Here's how the part is built. I have some questions about the finished solid (model axes, mm). A direction names the side the tool comes from. Give positions to 0.01 mm unless a question says otherwise; leave off trailing zeros. Loops run counter-clockwise (first coordinate to the right, second up) from the corner with the lowest first, then second, coordinate; pieces in that order, holes last. Notation, with made-up numbers: (16.5, 14.25) - (63.5, 14.25) arc R23 ccw to (63.5, 37.25) - close; hole circle Ø11 at (13, 53.25). An arc over 180 degrees is marked (long way). Use a Markdown table: item, result.
from build123d import *

# Parameters (mm, degrees)
SKETCH_1_W                         = 560
SKETCH_1_H                         = 90
SM_BASE_FLANGE_1_DEPTH             = 3
SM_EDGE_FLANGE_4_DEPTH             = 560
SM_START                           = 3
SM_EDGE_FLANGE_4_FLAT_DEPTH        = 3
SM_EDGE_FLANGE_4_BEND_DEPTH        = 560
SM_EDGE_FLANGE_4_FLAT_2_DEPTH      = 3
SM_EDGE_FLANGE_5_STRIP_W           = 13.4732
SM_EDGE_FLANGE_5_STRIP_H           = 3
SM_EDGE_FLANGE_5_STRIP_CUT_DEPTH   = 460
SM_EDGE_FLANGE_5_STRIP_2_W         = 13.4732
SM_EDGE_FLANGE_5_STRIP_2_H         = 3
SM_EDGE_FLANGE_5_STRIP_CUT_2_DEPTH = 460
SM_EDGE_FLANGE_5_DEPTH             = 460
SM_EDGE_FLANGE_5_BEND_DEPTH        = 460
FILLET_2_R                         = 5
HOLE_WIZARD_M6_1_D                 = 5
HOLE_WIZARD_M6_1_DEPTH             = 3
HOLE_WIZARD_M6_1_2_D               = 6.6
HOLE_WIZARD_M6_1_2_DEPTH           = 3
SKETCH_62_R                        = 10
SKETCH_62_R_2                      = 6
CUT_EXTRUDE_1_DEPTH                = 10
FILLET_3_R                         = 3
HOLE_WIZARD_M8_1_D                 = 9
SM_START_2                         = -44.7366
SM_EDGE_FLANGE_6_DEPTH             = 89.4732
SM_START_3                         = -45
SM_EDGE_FLANGE_6_2_DEPTH           = 90
SM_START_4                         = -283.7366
SM_EDGE_FLANGE_6_3_DEPTH           = 3
CUT_EXTRUDE_2_REACH                = 323.451
SKETCH_69_R                        = 6
CUT_EXTRUDE_3_REACH                = 333.07
FILLET_4_R                         = 3


with BuildPart() as part:
    # 베이스-플랜지1: sheet metal written as solids
    # Sketch 1 → 베이스-플랜지1 (new body)
    with BuildSketch(Plane(origin=(0, 0, 0), x_dir=(1, 0, 0), z_dir=(0, 1, 0))):
        Rectangle(SKETCH_1_W, SKETCH_1_H)
    extrude(amount=-SM_BASE_FLANGE_1_DEPTH)

    # 모서리 플랜지4: sheet metal written as solids
    # 모서리 플랜지4 bend section (on a plane across the edge) → 모서리 플랜지4 (add)
    with BuildSketch(Plane(origin=(-280, 0, 45.7366), x_dir=(0, 0, -1), z_dir=(1, 0, 0))):
        with BuildLine():
            Line((-3, 0.7366), (0, 0.7366))
            ThreePointArc((0, 0.7366), (0.215745145, 0.215745145), (0.7366, 0))
            Line((0.7366, 0), (0.7366, -3))
            ThreePointArc((0.7366, -3), (-1.905575199, -1.905575199), (-3, 0.7366))
        make_face()
    extrude(amount=SM_EDGE_FLANGE_4_DEPTH)

    # 모서리 플랜지4 profile (on flange) → 모서리 플랜지4 flat (add)
    with BuildSketch(Plane.XY.offset(45.7366).offset(SM_START)):
        Polygon((-280, 140), (-280, 0.7366), (280, 0.7366), (280, 20), (180, 20), (180, 140), align=None)
    extrude(amount=-SM_EDGE_FLANGE_4_FLAT_DEPTH)

    # 모서리 플랜지4 bend section 2 (on a plane across the edge) → 모서리 플랜지4 bend (add)
    with BuildSketch(Plane(origin=(280, 0, -45.7366), x_dir=(0, 0, 1), z_dir=(-1, 0, 0))):
        with BuildLine():
            Line((-3, 0.7366), (0, 0.7366))
            ThreePointArc((0, 0.7366), (0.215745145, 0.215745145), (0.7366, 0))
            Line((0.7366, 0), (0.7366, -3))
            ThreePointArc((0.7366, -3), (-1.905575199, -1.905575199), (-3, 0.7366))
        make_face()
    extrude(amount=SM_EDGE_FLANGE_4_BEND_DEPTH)

    # 모서리 플랜지4 profile 2 (on flange) → 모서리 플랜지4 flat 2 (add)
    with BuildSketch(Plane(origin=(0, 0, -45.7366), x_dir=(-1, 0, 0), z_dir=(0, 0, -1)).offset(SM_START)):
        Polygon((-280, 20), (-280, 0.7366), (280, 0.7366), (280, 140), (-180, 140), (-180, 20), align=None)
    extrude(amount=-SM_EDGE_FLANGE_4_FLAT_2_DEPTH)

    # 모서리 플랜지5: sheet metal written as solids
    # 모서리 플랜지5 strip (on a plane across the edge) → 모서리 플랜지5 strip cut (cut)
    with BuildSketch(Plane(origin=(-280, 140, 45.7366), x_dir=(0, -1, 0), z_dir=(1, 0, 0))):
        with Locations((-3, -1.5)):
            Rectangle(SM_EDGE_FLANGE_5_STRIP_W, SM_EDGE_FLANGE_5_STRIP_H)
    extrude(amount=SM_EDGE_FLANGE_5_STRIP_CUT_DEPTH, mode=Mode.SUBTRACT)

    # 모서리 플랜지5 strip 2 (on a plane across the edge) → 모서리 플랜지5 strip cut 2 (cut)
    with BuildSketch(Plane(origin=(180, 140, -45.7366), x_dir=(0, -1, 0), z_dir=(-1, 0, 0))):
        with Locations((-3, -1.5)):
            Rectangle(SM_EDGE_FLANGE_5_STRIP_2_W, SM_EDGE_FLANGE_5_STRIP_2_H)
    extrude(amount=SM_EDGE_FLANGE_5_STRIP_CUT_2_DEPTH, mode=Mode.SUBTRACT)

    # 모서리 플랜지5 section (on a plane across the edge) → 모서리 플랜지5 (add)
    with BuildSketch(Plane(origin=(-280, 140, 45.7366), x_dir=(0, -1, 0), z_dir=(1, 0, 0))):
        with BuildLine():
            Line((0, 0.7366), (0, 30))
            Line((0, 30), (3, 30))
            Line((3, 30), (3, 0.7366))
            ThreePointArc((3, 0.7366), (3.215745145, 0.215745145), (3.7366, 0))
            Line((3.7366, 0), (3.7366, -3))
            ThreePointArc((3.7366, -3), (1.094424801, -1.905575199), (0, 0.7366))
        make_face()
    extrude(amount=SM_EDGE_FLANGE_5_DEPTH)

    # 모서리 플랜지5 section 2 (on a plane across the edge) → 모서리 플랜지5 bend (add)
    with BuildSketch(Plane(origin=(180, 140, -45.7366), x_dir=(0, -1, 0), z_dir=(-1, 0, 0))):
        with BuildLine():
            Line((0, 0.7366), (0, 30))
            Line((0, 30), (3, 30))
            Line((3, 30), (3, 0.7366))
            ThreePointArc((3, 0.7366), (3.215745145, 0.215745145), (3.7366, 0))
            Line((3.7366, 0), (3.7366, -3))
            ThreePointArc((3.7366, -3), (1.094424801, -1.905575199), (0, 0.7366))
        make_face()
    extrude(amount=SM_EDGE_FLANGE_5_BEND_DEPTH)

    # 필렛2
    fillet_2_edges = [part.edges().sort_by_distance(p)[0] for p in [
        (280, 20, 47.2366),
        (280, 20, -47.2366),
    ]]
    fillet(fillet_2_edges, radius=FILLET_2_R)

    # Hole Wizard M6 _ _ _ _1
    with Locations(Plane(origin=(0, 140, 0), x_dir=(1, 0, 0), z_dir=(0, 1, 0))):
        with Locations((135, -30), (135, 30), (-65, 30), (-65, -30), (-265, -30), (-265, 30)):
            Hole(HOLE_WIZARD_M6_1_D / 2, depth=HOLE_WIZARD_M6_1_DEPTH)

    # Hole Wizard M6 _ _1 2
    with Locations(Plane(origin=(0, -3, 0), x_dir=(-1, 0, 0), z_dir=(0, -1, 0))):
        with Locations((90, -17.5), (90, 2.5), (230, -17.5), (230, 2.5), (-2.5, 7.5), (-2.5, -22.5), (-195, 27.5), (-220, 27.5), (-262.5, 5), (-262.5, -20)):
            Hole(HOLE_WIZARD_M6_1_2_D / 2, depth=HOLE_WIZARD_M6_1_2_DEPTH)

    # 스케치62 → 컷-돌출1 (cut)
    with BuildSketch(Plane(origin=(0, 140, 0), x_dir=(1, 0, 0), z_dir=(0, 1, 0))):
        with Locations((2.5, -22.5)):
            Circle(SKETCH_62_R)
        with Locations((-90, -17.5)):
            Circle(SKETCH_62_R_2)
        with Locations((-230, -17.5)):
            Circle(SKETCH_62_R_2)
        with Locations((132.5, -7.5)):
            Circle(SKETCH_62_R)
    extrude(amount=-CUT_EXTRUDE_1_DEPTH, mode=Mode.SUBTRACT)

    # 필렛3
    fillet_3_edges = [part.edges().sort_by_distance(p)[0] for p in [
        (-4.865895766, 138.5, 15.7366),
        (9.865895766, 138.5, 15.7366),
        (-95.735017039, 138.5, 15.7366),
        (-84.264982961, 138.5, 15.7366),
        (-235.735017039, 138.5, 15.7366),
        (-224.264982961, 138.5, 15.7366),
        (126.829160517, 138.5, 15.7366),
        (138.170839483, 138.5, 15.7366),
    ]]
    fillet(fillet_3_edges, radius=FILLET_3_R)

    # M8 여유 구멍1 (through all)
    with Locations(Plane(origin=(0, -3, 0), x_dir=(-1, 0, 0), z_dir=(0, -1, 0))):
        with Locations((-132.5, -7.5)):
            Hole(HOLE_WIZARD_M8_1_D / 2)

    # 모서리 플랜지6: read off the stored shape, not the designer's step
    # 모서리 플랜지6 outline → 모서리 플랜지6 (add)
    with BuildSketch(Plane.XY.offset(SM_START_2)):
        with BuildLine():
            Line((-280.7366, 140), (-283.7366, 140))
            Line((-283.7366, 140), (-283.7366, 0.7366))
            ThreePointArc((-283.7366, 0.7366), (-282.642175199, -1.905575199), (-280, -3))
            Line((-280, -3), (-280, 0))
            ThreePointArc((-280, 0), (-280.520854855, 0.215745145), (-280.7366, 0.7366))
            Line((-280.7366, 0.7366), (-280.7366, 140))
        make_face()
    extrude(amount=SM_EDGE_FLANGE_6_DEPTH)

    # Sm Edge Flange 6 2 outline → Sm Edge Flange 6 2 (add)
    with BuildSketch(Plane.XY.offset(SM_START_3)):
        with BuildLine():
            Line((-280.7366, 0.7366), (-283.7366, 0.7366))
            ThreePointArc((-283.7366, 0.7366), (-282.642175199, -1.905575199), (-280, -3))
            Line((-280, -3), (-280, 0))
            ThreePointArc((-280, 0), (-280.520854855, 0.215745145), (-280.7366, 0.7366))
        make_face()
    extrude(amount=SM_EDGE_FLANGE_6_2_DEPTH)

    # Sm Edge Flange 6 3 outline → Sm Edge Flange 6 3 (add)
    with BuildSketch(Plane.YZ.offset(SM_START_4)):
        with BuildLine():
            Line((0.7366, -48.7366), (136, -48.7366))
            ThreePointArc((136, -48.7366), (138.828427125, -47.565027125), (140, -44.7366))
            Line((140, -44.7366), (0.7366, -44.7366))
            Line((0.7366, -44.7366), (0.7366, -48.7366))
        make_face()
        with BuildLine():
            Line((136, 48.7366), (0.7366, 48.7366))
            Line((0.7366, 48.7366), (0.7366, 44.7366))
            Line((0.7366, 44.7366), (140, 44.7366))
            ThreePointArc((140, 44.7366), (138.828427125, 47.565027125), (136, 48.7366))
        make_face()
    extrude(amount=SM_EDGE_FLANGE_6_3_DEPTH)

    # 스케치69 → 컷-돌출2 (cut, up to next)
    with BuildSketch(Plane.XZ.offset(3), mode=Mode.PRIVATE) as cut_extrude_2_sk1:
        with Locations(Location((-105, 34, 0), (0, 0, 270))):
            Circle(SKETCH_69_R)
    cut_extrude_2_tool1 = extrude(cut_extrude_2_sk1.sketch, amount=-CUT_EXTRUDE_2_REACH, mode=Mode.PRIVATE) & part.part
    # 스케치69 → 컷-돌출2 (cut, up to next)
    with BuildSketch(Plane.XZ.offset(3), mode=Mode.PRIVATE) as cut_extrude_2_sk2:
        with Locations(Location((20, 34, 0), (0, 0, 270))):
            Circle(SKETCH_69_R)
    cut_extrude_2_tool2 = extrude(cut_extrude_2_sk2.sketch, amount=-CUT_EXTRUDE_2_REACH, mode=Mode.PRIVATE) & part.part
    # 스케치69 → 컷-돌출2 (cut, up to next)
    with BuildSketch(Plane.XZ.offset(3), mode=Mode.PRIVATE) as cut_extrude_2_sk3:
        with Locations(Location((160, -20, 0), (0, 0, 270))):
            Circle(SKETCH_69_R)
    cut_extrude_2_tool3 = extrude(cut_extrude_2_sk3.sketch, amount=-CUT_EXTRUDE_2_REACH, mode=Mode.PRIVATE) & part.part
    # 스케치69 → 컷-돌출2 (cut, up to next)
    with BuildSketch(Plane.XZ.offset(3), mode=Mode.PRIVATE) as cut_extrude_2_sk4:
        with BuildLine():
            Line((-244, 12.5), (-244, 2.5))
            ThreePointArc((-244, 2.5), (-250, -3.5), (-256, 2.5))
            Line((-256, 2.5), (-256, 12.5))
            ThreePointArc((-256, 12.5), (-250, 18.5), (-244, 12.5))
        make_face()
    cut_extrude_2_tool4 = extrude(cut_extrude_2_sk4.sketch, amount=-CUT_EXTRUDE_2_REACH, mode=Mode.PRIVATE) & part.part
    add(cut_extrude_2_tool1.solids().sort_by_distance((-105, -3, 34))[0], mode=Mode.SUBTRACT)
    add(cut_extrude_2_tool2.solids().sort_by_distance((20, -3, 34))[0], mode=Mode.SUBTRACT)
    add(cut_extrude_2_tool3.solids().sort_by_distance((160, -3, -20))[0], mode=Mode.SUBTRACT)
    add(cut_extrude_2_tool4.solids().sort_by_distance((-250, -3, 7.5))[0], mode=Mode.SUBTRACT)

    # 스케치70 → 컷-돌출3 (cut, up to next)
    with BuildSketch(Plane(origin=(0, 0, -48.7366), x_dir=(-1, 0, 0), z_dir=(0, 0, -1)), mode=Mode.PRIVATE) as cut_extrude_3_sk1:
        with BuildLine():
            Line((-75, 47), (-105, 47))
            ThreePointArc((-105, 47), (-113, 55), (-105, 63))
            Line((-105, 63), (-75, 63))
            ThreePointArc((-75, 63), (-67, 55), (-75, 47))
        make_face()
    cut_extrude_3_tool1 = extrude(cut_extrude_3_sk1.sketch, amount=-CUT_EXTRUDE_3_REACH, mode=Mode.PRIVATE) & part.part
    add(cut_extrude_3_tool1.solids().sort_by_distance((90, 55, -48.7366))[0], mode=Mode.SUBTRACT)

    # 필렛4
    fillet_4_edges = [part.edges().sort_by_distance(p)[0] for p in [
        (180, 138.5, -15.7366),
        (180, 138.5, 15.7366),
    ]]
    fillet(fillet_4_edges, radius=FILLET_4_R)


solid = part.part
(1) Will these pins go through, and if not, where does the flat tip stop? pin 1 (4 mm diameter, centred on y = 59.5, z = 2.5, fed in from +X); pin 2 (12 mm diameter, centred on x = 2.5, z = 22.5, fed in from +Y); pin 3 (2.5 mm diameter, centred on x = 91.5, y = 138.5, fed in from -Z).
A:
| item | result |
|---|---|
| pin 1 | x = -280.74 |
| pin 2 | y = 0 |
| pin 3 | z = -48.6 |
(2) Suppose I cut it at B-B on x = -153.5. Write out the boundary of the cut face in (y, z), plus the area to 3 significant figures.
A:
| item | result |
|---|---|
| outline | (-3, -45) arc R3.74 ccw to (0.74, -48.74) - (136.26, -48.74) arc R3.74 ccw to (140, -45) - (140, -15.74) - (137, -15.74) - (137, -45) arc R0.74 cw to (136.26, -45.74) - (0.74, -45.74) arc R0.74 cw to (0, -45) - (0, 45) arc R0.74 cw to (0.74, 45.74) - (136.26, 45.74) arc R0.74 cw to (137, 45) - (137, 15.74) - (140, 15.74) - (140, 45) arc R3.74 ccw to (136.26, 48.74) - (0.74, 48.74) arc R3.74 ccw to (-3, 45) - close |
| area | 1,300 mm2 |
(3) Suppose I cut it at A-A on y = 32. Write out the boundary of the cut face in (x, z).
A:
| item | result |
|---|---|
| outline | (-283.74, -48.74) - (-280.74, -48.74) - (-280.74, 48.74) - (-283.74, 48.74) - close; (-280, -48.74) - (180, -48.74) - (180, -45.74) - (-280, -45.74) - close; (-280, 45.74) - (180, 45.74) - (180, 48.74) - (-280, 48.74) - close |
(4) We'd pull the mould along X, two halves only. Please class faces 1 (the face through (20, -2, 40)), 2 (the face through (-280, 84, 47)), 3 (the face through (-283.737, 69, 1)), 4 (the face through (-4, -3, -1)): pulls with the +X half, pulls with the -X half, needs draft (parallel to the pull), parting line crosses it, or undercut.
A:
| item | result |
|---|---|
| face 1 | undercut |
| face 2 | undercut |
| face 3 | pulls with the -X half |
| face 4 | needs draft |
(5) If I drill on line 1 (X direction, y = 139.35, z = -30); line 2 (X direction, y = 138.65, z = 22.5); line 3 (Y direction, x = 144, z = 26), over which ranges is the centre line in solid material (lowest first)?
A:
| item | result |
|---|---|
| line 1 | -283.74 to -280.74, -280 to -267.5, -262.5 to -67.5, -62.5 to 132.5, 137.5 to 180 |
| line 2 | -283.74 to -280.74, -280 to -233.32, -226.68 to -93.32, -86.68 to -7.5, 12.5 to 180 |
| line 3 | -3 to 0, 137 to 140 |
(6) On a 3-axis mill with a long thin cutter (end or side, diameter ignored), from which of +Z, -Z, +X, -X, +Y, -Y can I reach the whole of each face in a straight line? I mean faces 5 (the face through (-66, 69, 45.737)), 6 (the face through (2.239, 138.521, 32.497)), 7 (the face through (180, 93, -46)), 8 (the face through (154.143, -1.521, -18.699)). Say none if no direction works.
A:
| item | result |
|---|---|
| face 5 | +X |
| face 6 | +Y |
| face 7 | +Z, -Z, +X, +Y |
| face 8 | -Y |
